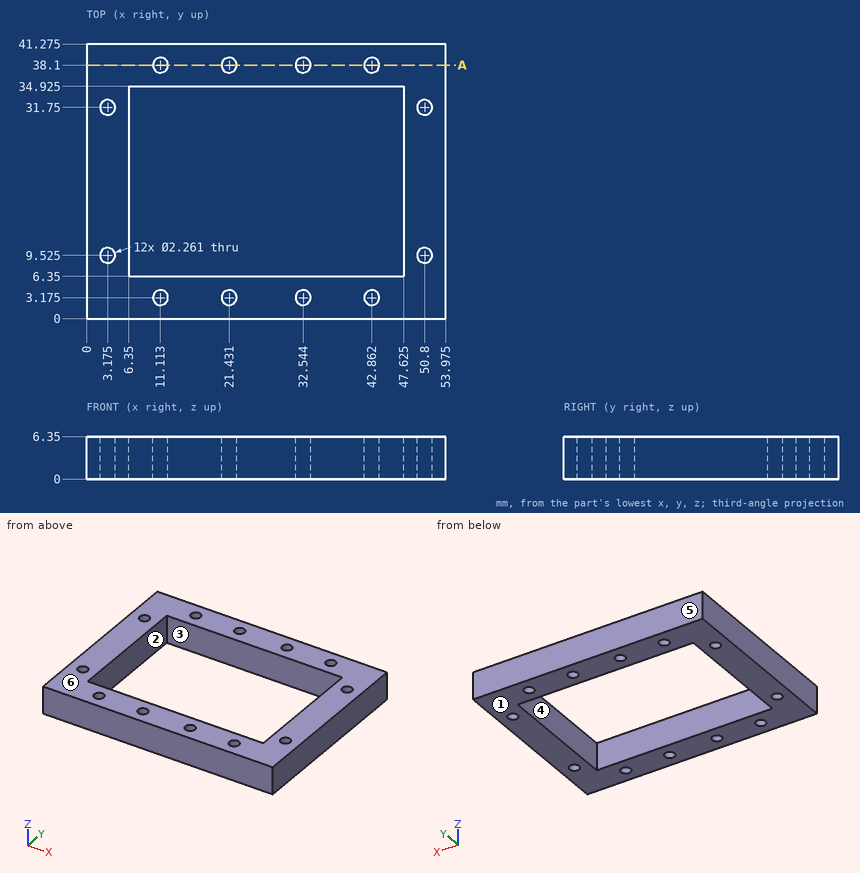
Check sheet for the drawn part. Datum: minimum x, y, z corner. Units: mm. A direction names the side the tool comes from. Give positions to 0.01 mm unless a question says otherwise; leave off trailing zeros. Answer as CSV lines item,"result".
Item 1: Set-up check for the marked faces 1 and 2: record each of +Z, -Z, +X, -X, +Y, -Y from which the full face is reachable in a straight line by a thin tool's end or side.
Reply:
face 1,"-Z, +X, -X, +Y, -Y"
face 2,"+Z, -Z"
Item 2: Draft check along Y on the marked faces 3, 4, 5 and 6. Enter one of: pulls with the +Y half, pulls with the -Y half, needs draft (parallel to the pull), parting line crosses it, or undercut.
Reply:
face 3,"undercut"
face 4,"undercut"
face 5,"pulls with the +Y half"
face 6,"needs draft"
Item 3: Scan lines: L1, parallel to Y at x = 50.8, z = 4 (1 decimal); L2, parallel to X at y = 4, z = 2 (1 decimal). Record each from-to range of solid material in increasing order.
Reply:
L1,"0 to 8.4, 10.7 to 30.6, 32.9 to 41.3"
L2,"0 to 10.3, 11.9 to 20.7, 22.2 to 31.8, 33.3 to 42.1, 43.6 to 54"
Item 4: Sectioned sample at A-A, the plane y = 38.1. State how many separate pieces and enclosed holes the cut face has, then the cut area to 3 significant figures.
Reply:
separate pieces,"5"
enclosed holes,"0"
area,"285 mm^2"
